Check sheet for the modelled part. Datum: model origin and axes. Units: mm. A direction names the side the tool comes from. Round coordinates to 2 decimals unless told otherwise and drop trailing zeros. Write each loop counter-clockwise with the first axis right and the second up, starting at its lowest first coordinate (ties: lowest second). Pieces come first, ordered by that corner, then holes. Notation, with made-up numbers: M -18.75,1 L 10.25,1 A27 cw 10.25,22 Z; hole C 57.25,75 d10. An arc over 180 degrees is marked long. One line per item, written item: value.
from build123d import *

# Parameters (mm, degrees)
SKETCH1_W           = 28.95
SKETCH1_H           = 64
SKETCH1_R           = 2
SKETCH1_R_2         = 4
BOSS_EXTRUDE1_DEPTH = 3
SKETCH2_R           = 1.6
BOSS_EXTRUDE2_DEPTH = 3
RIB1_REACH          = 75.226
SKETCH3_WALL_W      = 203.062325646
SKETCH3_WALL_H      = 3
RIB2_REACH          = 75.416
SKETCH4_WALL_W      = 203.442532142
SKETCH4_WALL_H      = 3


with BuildPart() as part:
    # Sketch1 → Boss-Extrude1 (new body)
    with BuildSketch(Plane(origin=(0, 0, 0), x_dir=(1, 0, 0), z_dir=(0, 1, 0))):
        with Locations((1.525, 0)):
            Rectangle(SKETCH1_W, SKETCH1_H)
        with Locations(Location((0, -24, 0), (0, 0, 270))):
            Circle(SKETCH1_R, mode=Mode.SUBTRACT)
        with Locations(Location((0, 24, 0), (0, 0, 270))):
            Circle(SKETCH1_R, mode=Mode.SUBTRACT)
        with Locations((0, 16)):
            Circle(SKETCH1_R_2, mode=Mode.SUBTRACT)
        with Locations(Location((0, -8, 0), (0, 0, 270))):
            Circle(SKETCH1_R, mode=Mode.SUBTRACT)
        with Locations(Location((8, 0, 0), (0, 0, 270))):
            Circle(SKETCH1_R, mode=Mode.SUBTRACT)
        with Locations(Location((0, 8, 0), (0, 0, 270))):
            Circle(SKETCH1_R, mode=Mode.SUBTRACT)
        with Locations(Location((0, 0, 0), (0, 0, 270))):
            Circle(SKETCH1_R_2, mode=Mode.SUBTRACT)
        with Locations((0, -16)):
            Circle(SKETCH1_R_2, mode=Mode.SUBTRACT)
        with Locations((0, -16)):
            Circle(SKETCH1_R_2)
        with Locations((0, 16)):
            Circle(SKETCH1_R_2)
    extrude(amount=BOSS_EXTRUDE1_DEPTH)

    # Sketch2 → Boss-Extrude2 (add)
    with BuildSketch(Plane.ZY.offset(12.95)):
        with BuildLine():
            Line((18, 51.05), (18, 12.95))
            ThreePointArc((18, 12.95), (20.914287527, 5.914287527), (27.95, 3))
            Line((27.95, 3), (32, 3))
            Line((32, 3), (32, 0))
            Line((32, 0), (-32, 0))
            Line((-32, 0), (-32, 3))
            Line((-32, 3), (-28.228, 3))
            ThreePointArc((-28.228, 3), (-21.192287527, 5.914287527), (-18.278, 12.95))
            Line((-18.278, 12.95), (-18.278, 51.05))
            Line((-18.278, 51.05), (18, 51.05))
        make_face()
        with Locations((-8.548, 48)):
            Circle(SKETCH2_R, mode=Mode.SUBTRACT)
        with Locations((-8.548, 16)):
            Circle(SKETCH2_R, mode=Mode.SUBTRACT)
        with Locations((7.452, 16)):
            Circle(SKETCH2_R, mode=Mode.SUBTRACT)
        with Locations((7.452, 48)):
            Circle(SKETCH2_R, mode=Mode.SUBTRACT)
    extrude(amount=-BOSS_EXTRUDE2_DEPTH)

    # Sketch3 wall → Rib1 (add, up to next)
    with BuildSketch(Plane(origin=(3.025, 27.025, 18), x_dir=(0.475191447028, -0.879882428891, 0), z_dir=(0.879882428891, 0.475191447028, 0)), mode=Mode.PRIVATE) as rib1_sk1:
        with Locations((0, 1.5)):
            Rectangle(SKETCH3_WALL_W, SKETCH3_WALL_H)
    rib1_tool1 = extrude(rib1_sk1.sketch, amount=-RIB1_REACH, mode=Mode.PRIVATE) - part.part
    add(rib1_tool1.solids().sort_by_distance((3.025, 27.025, 18))[0])

    # Sketch4 wall → Rib2 (add, up to next)
    with BuildSketch(Plane(origin=(3.025, 27.025, -18.278), x_dir=(0.475191447028, -0.879882428891, 0), z_dir=(-0.879882428891, -0.475191447028, 0)), mode=Mode.PRIVATE) as rib2_sk1:
        with Locations((0, 1.5)):
            Rectangle(SKETCH4_WALL_W, SKETCH4_WALL_H)
    rib2_tool1 = extrude(rib2_sk1.sketch, amount=RIB2_REACH, mode=Mode.PRIVATE) - part.part
    add(rib2_tool1.solids().sort_by_distance((3.025, 27.025, -18.278))[0])


solid = part.part
Q1. Sectioned sample at D-D on x = 7.25. Enter the section's corners in (y, z), and give its area (3 significant figures).
Completed:
outline: M 0,-32 L 3,-32 L 3,-18.28 L 19.2,-18.28 L 19.2,-15.28 L 3,-15.28 L 3,-1.85 L 0,-1.85 Z; M 0,1.85 L 3,1.85 L 3,15 L 19.2,15 L 19.2,18 L 3,18 L 3,32 L 0,32 Z
area: 278 mm^2
Q2. Sectioned sample at C-C on x = 0. State how many separate pieces and enclosed holes the cut face has, and give its area (3 significant figures).
Completed:
separate pieces: 6
enclosed holes: 0
area: 298 mm^2
Q3. Sectioned sample at B-B on y = 48. Enter the section's corners in (x, z), and give its area (3 significant figures).
Completed:
outline: M -12.95,-18.28 L -8.3,-18.28 L -8.3,-15.28 L -9.95,-15.28 L -9.95,-10.15 L -12.95,-10.15 Z; M -12.95,-6.95 L -9.95,-6.95 L -9.95,5.85 L -12.95,5.85 Z; M -12.95,9.05 L -9.95,9.05 L -9.95,15 L -8.3,15 L -8.3,18 L -12.95,18 Z
area: 99.5 mm^2
Q4. Sectioned sample at A-A on z = -23. Enter the section's corners in (x, y).
Completed:
outline: M -12.95,0 L -1.73,0 L -1.73,3 L -9.95,3 L -9.95,4.48 L -12.95,4.48 Z; M 1.73,0 L 16,0 L 16,3 L 1.73,3 Z
Q5. Depth check by flat-ended pin: P1, Ø8.5, axis at x = 3, y = 19, coming from the +Z side; P2, Ø6.5, axis at x = 0, z = 24, coming from the +Y side; P3, Ø4, axis at x = -5, y = 30.5, coming from the -Z side; P4, Ø1, axis at x = -3.5, z = 22, coming from the -Y side. Enter the tip coordinate at first touch or a pass-through.
Completed:
P1: z = 18
P2: y = 3
P3: z = -18.28
P4: y = 0
Q6. Draft check along Z on faces 5 (the cylindrical face through (-11.47, 5.99, 20.84)), 6 (the cylindrical face through (-3.905, 1.479, -0.867)), 7 (the flat face through (2.843, 27.361, -16.757)), 8 (the cylindrical face through (-11.471, 17.586, 7.244)). Enter one of: pulls with the +Z half, pulls with the -Z half, needs draft (parallel to the pull), parting line crosses it, or undercut.
Completed:
face 5: pulls with the +Z half
face 6: undercut
face 7: needs draft
face 8: undercut
Q7. Scan lines: line 1 (Z direction, x = -4.5, y = 15.5); line 2 (X direction, y = 0.8, z = -24); line 3 (Y direction, x = -2, z = 7.5). Record each from-to range of solid material in increasing order. Write a range as [from, to].
Completed:
line 1: [-18.28, -15.28], [15, 18]
line 2: [-12.95, -2], [2, 16]
line 3: [0, 3]
Q8. Access from +Z, -Z, +X, -X, +Y, -Y to the whole of each face (thin tool, end or side, straight path). Record for faces 1 (the flat face through (1, 3, 26)), 2 (the flat face through (1, 1, -32)), 3 (the flat face through (-2, 18, -18.278)), 4 (the flat face through (-9.95, 27, 0)).
Completed:
face 1: +Z, +X, +Y
face 2: -Z, +X, -X, +Y, -Y
face 3: -Z, +X, +Y
face 4: +X, +Y
